Read the model definition and answer for the solid it produces. Units are mm, in the model's axes. Face numbers are marked on the shaded views. Coordinates: 2 decimals unless noted, no trailing zeros. Write each loop counter-clockwise with the first axis right and the second up, starting at its lowest first coordinate (ties: lowest second). Pieces come first, ordered by that corner, then holes. Notation, with made-up numbers: (63.25, 56.5) -> (122.25, 56.5) arc R7 cw to (122.25, 62.5) -> close; hole circle Ø9 at (86, -31.75). An arc over 180 degrees is marked (long way). Answer in a Markdown table with one row per item. Add a question column.
Item 1: Section C-C on z = 1.95 is taken. Write down the section's boundary in (x, y), then the cut area to 3 significant figures.
Item 2: Section D-D on x = 18.5 is taken. Write down the section's boundary in (y, z), then the cut area to 3 significant figures.
Item 3: Section A-A on y = -5.75 is taken. Write down the section's boundary in (x, z), then the cut area to 3 significant figures.
Item 4: Straight lines are drawn through the part: line 1 (Y direction, x = 31, z = 1.05); line 2 (Y direction, x = 0, z = 1.95); line 3 (X direction, y = -0.75, z = 2.2). For each, find the intervals that lie inside material, in ascending order. Write a range as from..to.
Item 5: For a pull along X with two mould halves and no side action, classify the marked faces 1, 2 and 3 as +X half, -X half, draft (parallel to the pull), parting line (faces both ways), or undercut.
Item 6: Given pin 1 Ø6.5 at (x, y) = (0, 0) entering from +Z, flat-ended and moving along its own axis, determine where the tip first touches the part or whether it passes through.
Item 7: Section B-B on x = -0.5 is taken. Write down the section's boundary in (y, z), then the cut area to 3 significant figures.
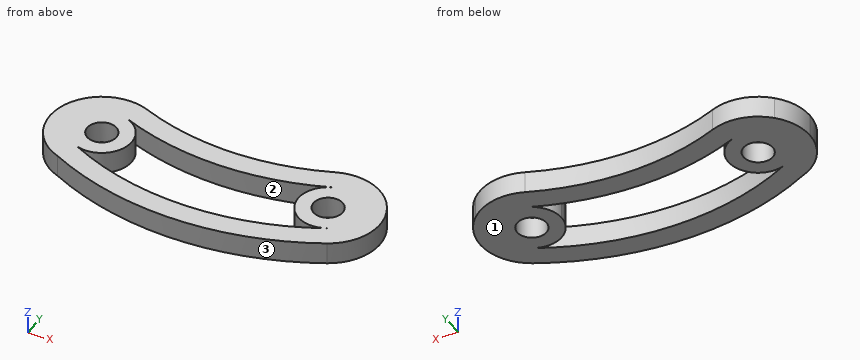
```python
from build123d import *

# Parameters (mm, degrees)
SKETCH1_R           = 1.5
EXTRUDE1_DEPTH      = 3
BOSS_EXTRUDE2_START = -3
BOSS_EXTRUDE2_DEPTH = 3
CUT_EXTRUDE4_START  = -5
CUT_EXTRUDE4_DEPTH  = 5
BOSS_EXTRUDE3_DEPTH = 3
BOSS_EXTRUDE4_DEPTH = 3
SKETCH7_R           = 2
CUT_EXTRUDE6_DEPTH  = 5


with BuildPart() as part:
    # Sketch1 → Extrude1 (new body)
    with BuildSketch(Plane.XY):
        with BuildLine():
            Line((0, -5), (31, -5))
            ThreePointArc((31, -5), (36, 0), (31, 5))
            Line((31, 5), (0, 5))
            ThreePointArc((0, 5), (-5, 0), (0, -5))
        make_face()
        with Locations((31, 0)):
            Circle(SKETCH1_R, mode=Mode.SUBTRACT)
        Circle(SKETCH1_R, mode=Mode.SUBTRACT)
    extrude(amount=EXTRUDE1_DEPTH)

    # Sketch2 → Boss-Extrude2 (add)
    with BuildSketch(Plane.XY.offset(3).offset(BOSS_EXTRUDE2_START)):
        with BuildLine():
            ThreePointArc((36, 0), (36, 5), (31, 5))
            ThreePointArc((31, 5), (34.535533906, 3.535533906), (36, 0))
        make_face()
        with BuildLine():
            Line((30.833786225, -5), (15.5, -5))
            Line((15.5, -5), (15.5, -10))
            ThreePointArc((15.5, -10), (23.564195558, -8.718430153), (30.833786225, -5))
        make_face()
        with BuildLine():
            Line((15.5, -10), (15.5, -5))
            Line((15.5, -5), (0.166213775, -5))
            ThreePointArc((0.166213775, -5), (7.435804442, -8.718430153), (15.5, -10))
        make_face()
        with BuildLine():
            ThreePointArc((-5, 0), (-3.535533906, 3.535533906), (0, 5))
            ThreePointArc((0, 5), (-5, 5), (-5, 0))
        make_face()
    extrude(amount=BOSS_EXTRUDE2_DEPTH)

    # Sketch2_6 → Cut-Extrude4 (cut)
    with BuildSketch(Plane.XY.offset(3).offset(CUT_EXTRUDE4_START)):
        with BuildLine():
            ThreePointArc((31, -5), (34.535533906, -3.535533906), (36, 0))
            ThreePointArc((36, 0), (33.590468728, -2.679345747), (30.833786225, -5))
            Line((30.833786225, -5), (31, -5))
        make_face()
        with BuildLine():
            ThreePointArc((0.166213775, -5), (-2.590468728, -2.679345747), (-5, 0))
            ThreePointArc((-5, 0), (-3.535533906, -3.535533906), (0, -5))
            Line((0, -5), (0.166213775, -5))
        make_face()
        with BuildLine():
            Line((31, 5), (15.5, 5))
            Line((15.5, 5), (15.5, -1.27314911))
            ThreePointArc((15.5, -1.27314911), (23.860657865, 0.354582479), (31, 5))
        make_face()
        with BuildLine():
            Line((15.5, -1.27314911), (15.5, 5))
            Line((15.5, 5), (0, 5))
            ThreePointArc((0, 5), (7.139342135, 0.354582479), (15.5, -1.27314911))
        make_face()
    extrude(amount=CUT_EXTRUDE4_DEPTH, mode=Mode.SUBTRACT)

    # Sketch5 → Boss-Extrude3 (add)
    with BuildSketch(Plane(origin=(0, 0, 0), x_dir=(-1, 0, 0), z_dir=(0, 0, -1))):
        with BuildLine():
            ThreePointArc((-31, 5), (-27.689986171, 2.356284055), (-23.93951242, 0.386671862))
            ThreePointArc((-23.93951242, 0.386671862), (-28.473717899, 6.604384812), (-36.000000042, 4.999999958))
            ThreePointArc((-36.000000042, 4.999999958), (-33.500000029, 6.035533906), (-31, 5))
        make_face()
        with BuildLine():
            ThreePointArc((-36.000000042, 4.999999958), (-36.911032421, -3.880682377), (-28.400293042, -6.575828749))
            ThreePointArc((-28.400293042, -6.575828749), (-32.520730735, -3.658414607), (-36, 0))
            ThreePointArc((-36, 0), (-37.035533906, 2.499999971), (-36.000000042, 4.999999958))
        make_face()
        with BuildLine():
            ThreePointArc((0, 5), (2.499999989, 6.035533906), (4.999999984, 5.000000016))
            ThreePointArc((4.999999984, 5.000000016), (-2.526282139, 6.604384797), (-7.06048758, 0.386671862))
            ThreePointArc((-7.06048758, 0.386671862), (-3.310013829, 2.356284055), (0, 5))
        make_face()
        with BuildLine():
            ThreePointArc((-2.599706958, -6.575828749), (3.976009043, -5.84733718), (7.071067812, 0))
            ThreePointArc((7.071067812, 0), (6.53281482, 2.705980511), (4.999999984, 5.000000016))
            ThreePointArc((4.999999984, 5.000000016), (6.035533906, 2.500000011), (5, 0))
            ThreePointArc((5, 0), (1.520730735, -3.658414607), (-2.599706958, -6.575828749))
        make_face()
    extrude(amount=-BOSS_EXTRUDE3_DEPTH)

    # Sketch6 → Boss-Extrude4 (add)
    with BuildSketch(Plane(origin=(0, 0, 0), x_dir=(-1, 0, 0), z_dir=(0, 0, -1))):
        with BuildLine():
            ThreePointArc((-7.06048758, 0.386671862), (-5.748903613, 4.117050795), (-2.639524867, 6.559947292))
            ThreePointArc((-2.639524867, 6.559947292), (-15.5, 4.069630639), (-28.360475133, 6.559947292))
            ThreePointArc((-28.360475133, 6.559947292), (-25.251096387, 4.117050795), (-23.93951242, 0.386671862))
            ThreePointArc((-23.93951242, 0.386671862), (-15.5, -1.27314911), (-7.06048758, 0.386671862))
        make_face()
        with BuildLine():
            ThreePointArc((-34.288674296, -6.259762086), (-15.993644495, -10.877173454), (2.396097668, -6.652722448))
            ThreePointArc((2.396097668, -6.652722448), (-0.108822543, -7.070230382), (-2.599706958, -6.575828749))
            ThreePointArc((-2.599706958, -6.575828749), (-15.5, -10), (-28.400293042, -6.575828749))
            ThreePointArc((-28.400293042, -6.575828749), (-31.379003341, -7.060903375), (-34.288674296, -6.259762086))
        make_face()
    extrude(amount=-BOSS_EXTRUDE4_DEPTH)

    # Sketch7 → Cut-Extrude6 (cut)
    with BuildSketch(Plane(origin=(0, 0, 0), x_dir=(-1, 0, 0), z_dir=(0, 0, -1))):
        with BuildLine():
            ThreePointArc((-29.480330692, 3.776797363), (-27.626554437, 2.278916006), (-26.928932188, 0))
            ThreePointArc((-26.928932188, 0), (-28.894602064, -3.484378375), (-32.893407958, -3.603969954))
            ThreePointArc((-32.893407958, -3.603969954), (-15.863554262, -7.878266077), (1.233165938, -3.879806039))
            ThreePointArc((1.233165938, -3.879806039), (-3.83098094, -1.377380909), (-1.519669308, 3.776797363))
            ThreePointArc((-1.519669308, 3.776797363), (-15.5, 1.069630639), (-29.480330692, 3.776797363))
        make_face()
        with Locations((-31, 0)):
            Circle(SKETCH7_R)
        Circle(SKETCH7_R)
    extrude(amount=-CUT_EXTRUDE6_DEPTH, mode=Mode.SUBTRACT)


solid = part.part
```
Results below:
| question | item | result |
|---|---|---|
| 1 | outline | (-2.4, -6.65) arc R40.26 ccw to (34.29, -6.26) arc R7.07 ccw to (28.36, 6.56) arc R34.45 cw to (2.64, 6.56) arc R7.07 ccw (long way) to start; hole circle Ø4 at (0, 0); hole (-1.23, -3.88) arc R37.26 ccw to (32.89, -3.6) arc R4.07 cw (long way) to (29.48, 3.78) arc R37.45 cw to (1.52, 3.78) arc R4.07 cw to start; hole circle Ø4 at (31, 0) |
| 1 | area | 376 mm2 |
| 2 | outline | (-10.77, 0) -> (-7.76, 0) -> (-7.76, 3) -> (-10.77, 3) -> close; (1.19, 0) -> (4.2, 0) -> (4.2, 3) -> (1.19, 3) -> close |
| 2 | area | 18.1 mm2 |
| 3 | outline | (-4.12, 0) -> (3.15, 0) -> (3.15, 3) -> (-4.12, 3) -> close; (27.98, 0) -> (35.12, 0) -> (35.12, 3) -> (27.98, 3) -> close |
| 3 | area | 43.2 mm2 |
| 4 | line 1 | y = -7.8..-4.53, -4.07..-2, 2..7.07 |
| 4 | line 2 | y = -7.75..-4.47, -4.07..-2, 2..7.07 |
| 4 | line 3 | x = -7.03..-1.85, 1.85..4, 27..29.15, 32.85..38.03 |
| 5 | face 1 | draft |
| 5 | face 2 | undercut |
| 5 | face 3 | parting line |
| 6 | pin 1 | stops at z = 3 |
| 7 | outline | (-7.54, 0) -> (-4.24, 0) -> (-4.24, 3) -> (-7.54, 3) -> close; (-4.04, 0) -> (-1.94, 0) -> (-1.94, 3) -> (-4.04, 3) -> close; (1.94, 0) -> (7.05, 0) -> (7.05, 3) -> (1.94, 3) -> close |
| 7 | area | 31.6 mm2 |
